Read the model definition and answer for the solid it produces. Units are mm, in the model's axes. A direction names the side the tool comes from. Give positions to 0.01 mm unless a question says otherwise; leave off trailing zeros. Order: outer loops, then holes, each group sorted by start corner. A loop starts at its lowest first (then second) coordinate and runs counter-clockwise, first axis right, second up. Notation, with made-up numbers: (27.5, 76) - (61.5, 76) arc R20 ccw to (61.5, 108) - close; hole circle Ø10 at (-20, 0). An arc over 180 degrees is marked (long way). Return JSON: item names as keys, results as strings.
```python
from build123d import *

# Parameters (mm, degrees)
SKETCH2_W                = 30
SKETCH2_H                = 30
BOSS_EXTRUDE1_DEPTH      = 120
SKETCH5_R                = 3.4
CUT_EXTRUDE2_DEPTH       = 122.86057607
CUT_EXTRUDE1_DEPTH       = 122.86057607
FILLET1_R                = 2.5
FILLET2_R                = 0.3
CIRPATTERN1_COUNT        = 4
FILLET1_OF_CIRPATTERN1_R = 2.5
FILLET2_OF_CIRPATTERN1_R = 0.3


with BuildPart() as part:
    # Sketch2 → Boss-Extrude1 (new body)
    with BuildSketch(Plane(origin=(0, 0, 0), x_dir=(0, 0, -1), z_dir=(1, 0, 0))):
        Rectangle(SKETCH2_W, SKETCH2_H)
    extrude(amount=BOSS_EXTRUDE1_DEPTH)

    # Sketch5 → Cut-Extrude2 (cut, through all)
    with BuildSketch(Plane(origin=(120, 0, 0), x_dir=(0, 0, -1), z_dir=(1, 0, 0))):
        Circle(SKETCH5_R)
    extrude(amount=-CUT_EXTRUDE2_DEPTH, mode=Mode.SUBTRACT)

    # Sketch4 → Cut-Extrude1 (cut, through all)
    with BuildSketch(Plane(origin=(120, 0, 0), x_dir=(0, 0, -1), z_dir=(1, 0, 0))):
        with BuildLine():
            Line((-4.385786454, -5.8), (4.385786454, -5.8))
            Line((4.385786454, -5.8), (8.162132034, -9.57634558))
            ThreePointArc((8.162132034, -9.57634558), (8.22716386, -9.673672585), (8.25, -9.788477614))
            Line((8.25, -9.788477614), (8.25, -13))
            Line((8.25, -13), (4.1, -13))
            Line((4.1, -13), (4.1, -14))
            Line((4.1, -14), (5.1, -14))
            Line((5.1, -14), (5.1, -15))
            Line((5.1, -15), (-5.1, -15))
            Line((-5.1, -15), (-5.1, -14))
            Line((-5.1, -14), (-4.1, -14))
            Line((-4.1, -14), (-4.1, -13))
            Line((-4.1, -13), (-8.25, -13))
            Line((-8.25, -13), (-8.25, -9.788477614))
            ThreePointArc((-8.25, -9.788477614), (-8.22716386, -9.673672585), (-8.162132034, -9.57634558))
            Line((-8.162132034, -9.57634558), (-4.385786454, -5.8))
        make_face()
        with BuildLine():
            Line((11.05, -10.05), (12.65, -10.05))
            ThreePointArc((12.65, -10.05), (13.357106781, -10.342893219), (13.65, -11.05))
            Line((13.65, -11.05), (13.65, -12.65))
            ThreePointArc((13.65, -12.65), (13.357106781, -13.357106781), (12.65, -13.65))
            Line((12.65, -13.65), (11.05, -13.65))
            ThreePointArc((11.05, -13.65), (10.342893219, -13.357106781), (10.05, -12.65))
            Line((10.05, -12.65), (10.05, -11.05))
            ThreePointArc((10.05, -11.05), (10.342893219, -10.342893219), (11.05, -10.05))
        make_face()
        with BuildLine():
            Line((4.065863992, -3.00520382), (2.87527145, -1.814611278))
            ThreePointArc((2.87527145, -1.814611278), (2.404163056, -2.404163056), (1.814611278, -2.87527145))
            Line((1.814611278, -2.87527145), (3.00520382, -4.065863992))
            ThreePointArc((3.00520382, -4.065863992), (4.065863992, -4.065863992), (4.065863992, -3.00520382))
        make_face()
    cut_extrude1 = extrude(amount=-CUT_EXTRUDE1_DEPTH, mode=Mode.SUBTRACT)

    # Fillet1
    fillet1_edges = [part.edges().sort_by_distance(p)[0] for p in [
        (60, -15, -15),
    ]]
    fillet(fillet1_edges, radius=FILLET1_R)

    # Fillet2
    fillet2_edges = [part.edges().sort_by_distance(p)[0] for p in [
        (60, -13, -8.25),
        (60, -13, -4.1),
        (60, -14, -4.1),
        (60, -14, -5.1),
        (60, -15, -5.1),
        (60, -15, 5.1),
        (60, -14, 5.1),
        (60, -14, 4.1),
        (60, -13, 4.1),
        (60, -13, 8.25),
    ]]
    fillet(fillet2_edges, radius=FILLET2_R)

    # CirPattern1: Cut-Extrude1 ×4 about axis
    cirpattern1_axis = Axis((0, 0, 0), (1, 0, 0))
    for i in range(1, CIRPATTERN1_COUNT):
        add(cut_extrude1.rotate(cirpattern1_axis, i * 360 / CIRPATTERN1_COUNT), mode=Mode.SUBTRACT)

    # Fillet1 of CirPattern1
    fillet1_of_cirpattern1_edges = [part.edges().sort_by_distance(p)[0] for p in [
        (60, 15, -15),
        (60, 15, 15),
        (60, -15, 15),
    ]]
    fillet(fillet1_of_cirpattern1_edges, radius=FILLET1_OF_CIRPATTERN1_R)

    # Fillet2 of CirPattern1
    fillet2_of_cirpattern1_edges = [part.edges().sort_by_distance(p)[0] for p in [
        (60, 8.25, -13),
        (60, 4.1, -13),
        (60, 4.1, -14),
        (60, 5.1, -14),
        (60, 5.1, -15),
        (60, -5.1, -15),
        (60, -5.1, -14),
        (60, -4.1, -14),
        (60, -4.1, -13),
        (60, -8.25, -13),
        (60, 13, 8.25),
        (60, 13, 4.1),
        (60, 14, 4.1),
        (60, 14, 5.1),
        (60, 15, 5.1),
        (60, 15, -5.1),
        (60, 14, -5.1),
        (60, 14, -4.1),
        (60, 13, -4.1),
        (60, 13, -8.25),
        (60, -8.25, 13),
        (60, -4.1, 13),
        (60, -4.1, 14),
        (60, -5.1, 14),
        (60, -5.1, 15),
        (60, 5.1, 15),
        (60, 5.1, 14),
        (60, 4.1, 14),
        (60, 4.1, 13),
        (60, 8.25, 13),
    ]]
    fillet(fillet2_of_cirpattern1_edges, radius=FILLET2_OF_CIRPATTERN1_R)


solid = part.part
```
Q1. A cutting plane is placed at A-A (z = -0.25). Write down the section's boundary in (x, y).
Values:
{"outline": "(0, -5.8) - (120, -5.8) - (120, -3.39) - (0, -3.39) - close; (0, 3.39) - (120, 3.39) - (120, 5.8) - (0, 5.8) - close"}
Q2. For faces 1 (the flat face through (61, -11, 8.25)), 2 (the flat face through (59, -9, 15)), determine the directions among +Z, -Z, +X, -X, +Y, -Y from which every point of the face is accessible in a straight line to the end or side of a thin tool.
Values:
{"face 1": "+X, -X", "face 2": "+Z, +X, -X, +Y, -Y"}
Q3. A cutting plane is placed at C-C (x = 29). Give the number of separate pieces and of enclosed holes in the cut face, and give its area (3 significant figures).
Values:
{"separate pieces": "1", "enclosed holes": "5", "area": "307 mm²"}
Q4. Determine the mould class of faces 3 (the flat face through (59, 9, 15)), 4 (the flat face through (60.84, -7.715, 6.3)), 5 (the flat face through (61, 11, -8.25)), 6 (the flat face through (59, -15, -9)) for opening direction Y: released by +Y, released by -Y, zero draft, split by the parting line, or undercut.
Values:
{"face 3": "zero draft", "face 4": "undercut", "face 5": "undercut", "face 6": "released by -Y"}
Q5. Given pin 1 (1.5 mm diameter, centred on x = 87.5, z = -4, fed in from +Y), flat-ended and moving along its own axis, determine where the tip first touches the part or whether it passes through.
Values:
{"pin 1": "stops at y = 14"}
Q6. A cutting plane is placed at B-B (y = -0.5). Write down the section's boundary in (x, z), and give its area (3 significant figures).
Values:
{"outline": "(0, -5.8) - (120, -5.8) - (120, -3.36) - (0, -3.36) - close; (0, 3.36) - (120, 3.36) - (120, 5.8) - (0, 5.8) - close", "area": "585 mm²"}
Q7. Consider L1, parallel to Z at x = 105.5, y = 11.75. Determine where the line is inside the solid, lowest interval first.
Values:
{"L1": "z = -15 to -13.65, -10.05 to -8.25, 8.25 to 10.05, 13.65 to 15"}
